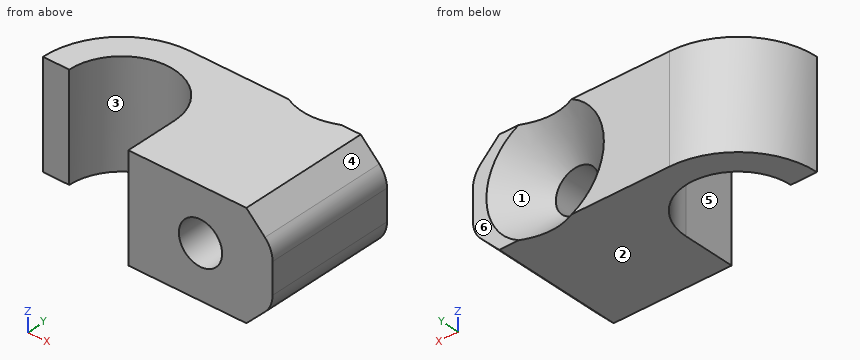
```python
from build123d import *

# Parameters (mm, degrees)
F1_DEPTH       = 4
F3_D           = 3.3
F3_CSINK_D     = 8.96
F3_CSINK_ANGLE = 90
F4_SIZE        = 2
F5_R           = 2


with BuildPart() as f1:
    # F0 (on Top) → F1 (new body, symmetric)
    with BuildSketch(Plane.XY):
        with BuildLine():
            ThreePointArc((-15.5993879735, 12.218022719), (-11.5993879735, 16.218022719), (-7.5993879735, 12.218022719))
            Line((-7.5993879735, 12.218022719), (-7.5993879735, 8.218022719))
            Line((-7.5993879735, 8.218022719), (3.4006120265, 8.218022719))
            Line((3.4006120265, 8.218022719), (3.4006120265, 18.218022719))
            Line((3.4006120265, 18.218022719), (-11.5993879735, 18.218022719))
            ThreePointArc((-11.5993879735, 18.218022719), (-15.8420286607, 16.4606634061), (-17.5993879735, 12.218022719))
            Line((-17.5993879735, 12.218022719), (-15.5993879735, 12.218022719))
        make_face()
    extrude(amount=F1_DEPTH, both=True)

    # F3 (through all)
    with Locations(Plane(origin=(0, 18.218022719, 0), x_dir=(-1, 0, 0), z_dir=(0, 1, 0))):
        with Locations((2.0993879735, 0)):
            CounterSinkHole(F3_D / 2, F3_CSINK_D / 2, counter_sink_angle=F3_CSINK_ANGLE)

    # F4
    f4_edges = [f1.edges().sort_by_distance(p)[0] for p in [
        (3.400612, 13.218023, 4),
        (3.400612, 13.218023, -4),
    ]]
    chamfer(f4_edges, length=F4_SIZE)

    # F5
    f5_edges = [f1.edges().sort_by_distance(p)[0] for p in [
        (3.400612, 13.218023, 2),
        (3.400612, 13.218023, -2),
    ]]
    fillet(f5_edges, radius=F5_R)


solid = f1.part
```
Part model, mm, in its own coordinate system. Face numbers are marked on the shaded views. A direction names the side the tool comes from. Round coordinates to 2 decimals unless told otherwise and drop trailing zeros. Write each loop counter-clockwise with the first axis right and the second up, starting at its lowest first coordinate (ties: lowest second). Pieces come first, ordered by that corner, then holes.
Item 1: Two-plate mould, pull along Z, no slides. Class the marked faces 1, 2, 3 and 4: +Z half, -Z half, draft (parallel to the pull), parting line (faces both ways), or undercut.
Results:
face 1: undercut
face 2: -Z half
face 3: draft
face 4: +Z half
Item 2: Cut at B-B, the plane y = 14.5. Give the cut face in (x, z), plus the area to 3 significant figures.
Results:
outline: (-17.15, -4) - (-14.88, -4) - (-14.88, 4) - (-17.15, 4) - close; (-8.31, -4) - (1.4, -4) - (2.81, -2.59) arc R2 ccw to (3.4, -1.17) - (3.4, 1.17) arc R2 ccw to (2.81, 2.59) - (1.4, 4) - (-8.31, 4) - close; hole circle Ø3.3 at (-2.1, 0)
area: 99.1 mm2
Item 3: Which spindle directions (+Z, -Z, +X, -X, +Y, -Y) get a long thin tool onto all of the face, cutting with end or side? Do the marked faces 5 and 6. Say none if no direction does.
Results:
face 5: +Z, -Z, -X, -Y
face 6: +Z, -Z, +X, -X, +Y
Item 4: Cut at D-D, the plane y = 13. Give the cut face in (x, z).
Results:
outline: (-17.55, -4) - (-15.52, -4) - (-15.52, 4) - (-17.55, 4) - close; (-7.68, -4) - (1.4, -4) - (2.81, -2.59) arc R2 ccw to (3.4, -1.17) - (3.4, 1.17) arc R2 ccw to (2.81, 2.59) - (1.4, 4) - (-7.68, 4) - close; hole circle Ø3.3 at (-2.1, 0)
Item 5: Cut at A-A, the plane y = 9.5. Give the cut face in (x, z), plus the area to 3 significant figures.
Results:
outline: (-7.6, -4) - (1.4, -4) - (2.81, -2.59) arc R2 ccw to (3.4, -1.17) - (3.4, 1.17) arc R2 ccw to (2.81, 2.59) - (1.4, 4) - (-7.6, 4) - close; hole circle Ø3.3 at (-2.1, 0)
area: 75.3 mm2
Item 6: Cut at C-C, the plane z = 0. Give the cut face in (x, y), plus the area to 3 significant figures.
Results:
outline: (-17.6, 12.22) - (-15.6, 12.22) arc R4 cw to (-7.6, 12.22) - (-7.6, 8.22) - (-3.75, 8.22) - (-3.75, 15.39) - (-6.58, 18.22) - (-11.6, 18.22) arc R6 ccw to start; (-0.45, 8.22) - (3.4, 8.22) - (3.4, 18.22) - (2.38, 18.22) - (-0.45, 15.39) - close
area: 96.1 mm2
Item 7: Drop flat-ended pins along their axis: pin 1 Ø4.5 at (y, z) = (9.5, 1) entering from -X; pin 2 Ø4.5 at (x, z) = (-2.1, 0) entering from +Y; pin 3 Ø1 at (x, z) = (-17, 0.5) entering from -Y. Give the stop position or say it passes through.
Results:
pin 1: stops at x = -7.6
pin 2: stops at y = 15.99
pin 3: stops at y = 12.22
Item 8: Probe L1, parallel to X at y = 9.75, z = 0; L2, parallel to X at y = 13, z = 0; L3, parallel to Y at x = -11.75, z = 2. List the from-to ranges inside material, lowest first.
Results:
L1: x = -7.6 to -3.75, -0.45 to 3.4
L2: x = -17.55 to -15.52, -7.68 to -3.75, -0.45 to 3.4
L3: y = 16.22 to 18.22
